Answer from the drawing. Dimensions are ordinates in mm from the lowest x, y and z of the part. A direction names the side the tool comes from. Coordinates: 2 decimals unless noted, no trailing zeros. Write each loop counter-clockwise with the first axis right and the second up, starting at its lowest first coordinate (ties: lowest second). Pieces come first, ordered by that corner, then holes.
(1) The part is cut by section C-C on z = 1.75. Determine the outline of the cut face in (x, y).
(2) For a pull along X with two mould halves and no side action, classify the marked faces 1, 2 and 3 as +X half, -X half, draft (parallel to the pull), parting line (faces both ways), or undercut.
(3) Which of the six approach directions +Z, -Z, +X, -X, +Y, -Y give full straight-line access (tool end or side, diameter ignored) to the marked faces 4, 5, 6, 7 and 8?
(4) The part is cut by section D-D on x = 29. Determine the outline of the cut face in (y, z), plus the area to 3 significant figures.
(5) The part is cut by section A-A on z = 6.35. Determine the outline of the cut face in (x, y).
(6) The part is cut by section B-B on y = 6.35. Determine the outline of the cut face in (x, z), plus the area to 3 significant figures.
(7) Straight lines are drawn through the part: line 1 (X direction, y = 4.5, z = 1); line 2 (Z direction, x = 54.95, y = 6.35); line 3 (Y direction, x = 24, z = 1.5). For each, find the intervals that lie inside material, in ascending order.
(8) Given P1, Ø4, axis at y = 6.5, z = 7, coming from the +X side; P2, Ø1.5, axis at x = 46, z = 11, coming from the -Y side; P3, Ø4, axis at y = 7.5, z = 6, coming from the -X side; P4, Ø2, axis at y = 6.35, z = 6.35, coming from the -X side, each flat-ended and moving along its own axis, determine where each tip first touches the part or whether it passes through.
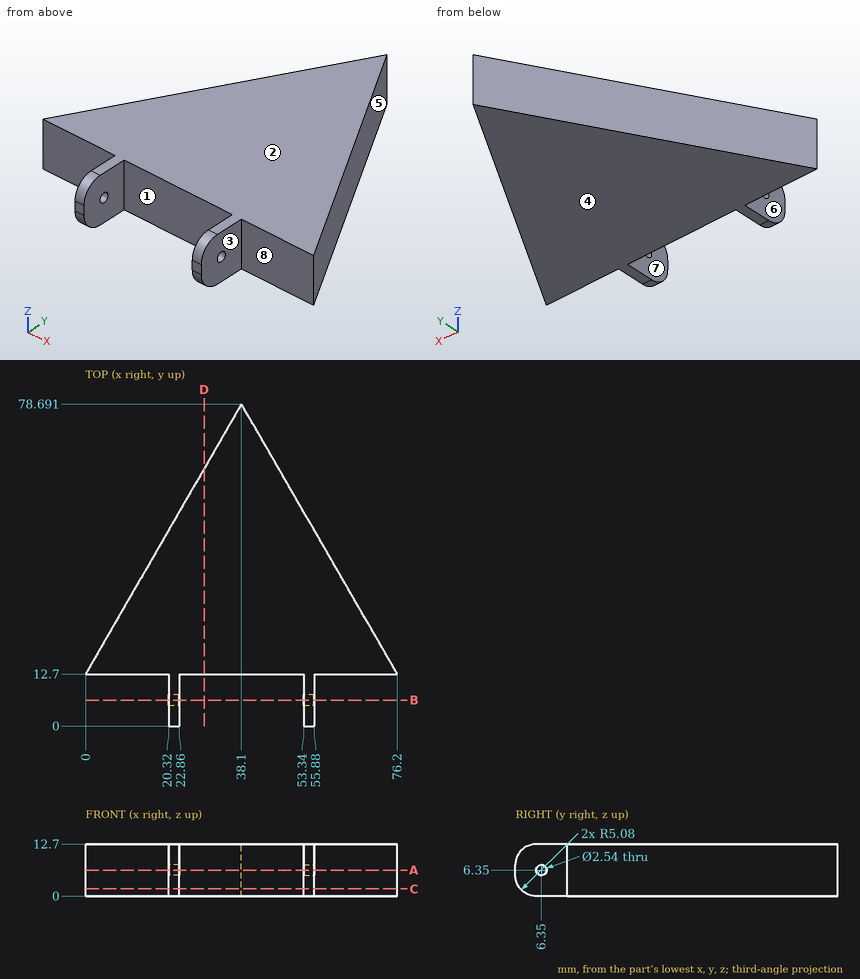
Model answer:
1. outline: (0, 12.7) - (20.32, 12.7) - (20.32, 1.24) - (22.86, 1.24) - (22.86, 12.7) - (53.34, 12.7) - (53.34, 1.24) - (55.88, 1.24) - (55.88, 12.7) - (76.2, 12.7) - (38.1, 78.69) - close
2. face 1: undercut
2. face 2: draft
2. face 3: +X half
3. face 4: -Z, +X, -X, +Y, -Y
3. face 5: +Z, -Z, +X, +Y
3. face 6: +Z, -Z, -X, -Y
3. face 7: +Z, -Z, -Y
3. face 8: +Z, -Z, +X, -Y
4. outline: (12.7, 0) - (62.93, 0) - (62.93, 12.7) - (12.7, 12.7) - close
4. area: 638 mm2
5. outline: (0, 12.7) - (20.32, 12.7) - (20.32, 7.62) - (22.86, 7.62) - (22.86, 12.7) - (53.34, 12.7) - (53.34, 7.62) - (55.88, 7.62) - (55.88, 12.7) - (76.2, 12.7) - (38.1, 78.69) - close; (20.32, 0) - (22.86, 0) - (22.86, 5.08) - (20.32, 5.08) - close; (53.34, 0) - (55.88, 0) - (55.88, 5.08) - (53.34, 5.08) - close
6. outline: (20.32, 0) - (22.86, 0) - (22.86, 5.08) - (20.32, 5.08) - close; (20.32, 7.62) - (22.86, 7.62) - (22.86, 12.7) - (20.32, 12.7) - close; (53.34, 0) - (55.88, 0) - (55.88, 5.08) - (53.34, 5.08) - close; (53.34, 7.62) - (55.88, 7.62) - (55.88, 12.7) - (53.34, 12.7) - close
6. area: 51.6 mm2
7. line 1: x = 20.32 to 22.86, 53.34 to 55.88
7. line 2: z = 0 to 5.08, 7.62 to 12.7
7. line 3: y = 12.7 to 54.27
8. P1: stops at x = 55.88
8. P2: stops at y = 12.7
8. P3: stops at x = 20.32
8. P4: passes through
